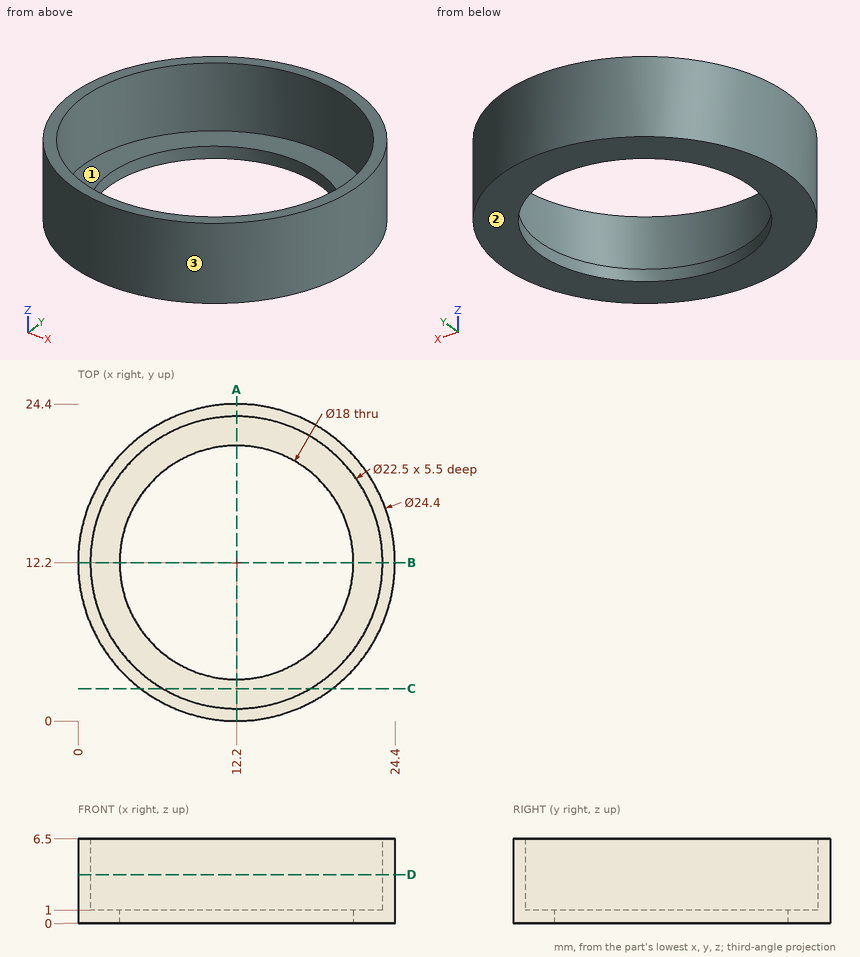
Part print with two shaded views. Sizes in mm from the minimum x, y, z corner. Round coordinates to 2 decimals unless told otherwise and drop trailing zeros. Order: outer loops, then holes, each group sorted by start corner. A loop starts at its lowest first (then second) coordinate and runs counter-clockwise, first axis right, second up. Notation, with made-up numbers: (81.5, 38.25) - (95.5, 38.25) arc R33 ccw to (95.5, 74.25) - close; hole circle Ø2 at (2, 59.5). An arc over 180 degrees is marked (long way). Return JSON: item names as keys, results as strings.
(1) Wall check: probe 1 along Y at (x, z) = (12.2, 0.35); probe 2 along Y at (x, z) = (12.2, 3.65); probe 3 along Z at (x, y) = (21, 8). Give the ranges that are in metal, low to high. Write a range as from..to.
Answer key:
{"probe 1": "y = 0..3.2, 21.2..24.4", "probe 2": "y = 0..0.95, 23.45..24.4", "probe 3": "z = 0..1"}
(2) Pull direction Y, two halves, no side cores. Call the marked faces 1, 2 and 3: +Y half, -Y half, draft (parallel to the pull), parting line (faces both ways), or undercut.
Answer key:
{"face 1": "undercut", "face 2": "draft", "face 3": "parting line"}
(3) Cut at D-D (z = 3.75). Give the cut face in (x, y).
Answer key:
{"outline": "circle Ø24.4 at (12.2, 12.2); hole circle Ø22.5 at (12.2, 12.2)"}
(4) Cut at A-A (x = 12.2). Give the cut face in (y, z), then the cut area to 4 significant figures.
Answer key:
{"outline": "(0, 0) - (3.2, 0) - (3.2, 1) - (0.95, 1) - (0.95, 6.5) - (0, 6.5) - close; (21.2, 0) - (24.4, 0) - (24.4, 6.5) - (23.45, 6.5) - (23.45, 1) - (21.2, 1) - close", "area": "16.85 mm^2"}
(5) Pin check, flat tips, straight feed: pin 1 Ø1 at (y, z) = (21.5, 2) entering from +X; pin 2 Ø12 at (x, y) = (14.5, 15.5) entering from +Z. Stop position of each tip, or through.
Answer key:
{"pin 1": "stops at x = 20.65", "pin 2": "stops at z = 1"}
(6) Cut at C-C (y = 2.5). Give the cut face in (x, z).
Answer key:
{"outline": "(4.8, 0) - (19.6, 0) - (19.6, 6.5) - (17.9, 6.5) - (17.9, 1) - (6.5, 1) - (6.5, 6.5) - (4.8, 6.5) - close"}
